Here's how the part is built. I have some questions about the finished solid (model axes, mm). Give positions to 0.01 mm unless a question says otherwise; leave off trailing zeros. Write each loop counter-clockwise with the first axis right and the second up, starting at its lowest first coordinate (ties: lowest second). Pieces come first, ordered by that corner, then holes. Notation, with made-up numbers: (33, 4) - (76, 4) arc R14 cw to (76, 24) - close; hole circle Ø8 at (39.25, -29). An arc over 180 degrees is marked (long way). One line per item, written item: value. Start each with the question number.
1) Imagine slicing it at A-A on z = 50. Write out the boundary of the cut face in (x, y), plus the area to 3 significant figures.
2) I'm going to push a flat-ended pin straight in: P1, Ø6, axis at x = -79.4, z = 50, coming from the +Y side. Where does the tip first touch, or does it pass through?
3) Imagine slicing it at B-B on x = 79.4. Write out the boundary of the cut face in (y, z), plus the area to 3 significant figures.
4) Please list where these lines run through material, in increasing order: L1, parallel to X at y = -4.5, z = 50; L2, parallel to Z at x = -79.4, y = -3.5. Write a range as [from, to].
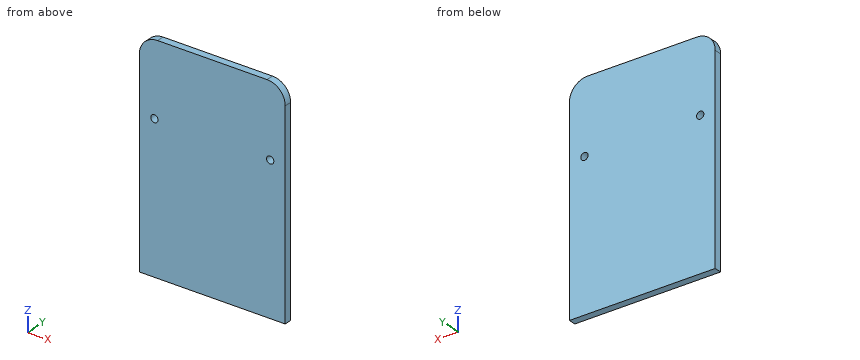
from build123d import *

# Parameters (mm, degrees)
BOSS_EXTRUDE1_DEPTH = 10
SKETCH2_R           = 5
CUT_EXTRUDE1_DEPTH  = 11


with BuildPart() as part:
    # Sketch1 → Boss-Extrude1 (new body)
    with BuildSketch(Plane(origin=(0, 0, 0), x_dir=(1, 0, 0), z_dir=(0, 1, 0))):
        with BuildLine():
            Line((-100, 150), (100, 150))
            Line((100, 150), (100, -125))
            ThreePointArc((100, -125), (92.67766953, -142.67766953), (75, -150))
            Line((75, -150), (-75, -150))
            ThreePointArc((-75, -150), (-92.67766953, -142.67766953), (-100, -125))
            Line((-100, -125), (-100, 150))
        make_face()
    extrude(amount=-BOSS_EXTRUDE1_DEPTH)

    # Sketch2 → Cut-Extrude1 (cut, through all)
    with BuildSketch(Plane(origin=(0, 0, 0), x_dir=(1, 0, 0), z_dir=(0, 1, 0))):
        with Locations((-79.4, -50)):
            Circle(SKETCH2_R)
        with Locations((79.4, -50)):
            Circle(SKETCH2_R)
    extrude(amount=-CUT_EXTRUDE1_DEPTH, mode=Mode.SUBTRACT)


solid = part.part
Numbers:
1. outline: (-100, -10) - (-84.4, -10) - (-84.4, 0) - (-100, 0) - close; (-74.4, -10) - (74.4, -10) - (74.4, 0) - (-74.4, 0) - close; (84.4, -10) - (100, -10) - (100, 0) - (84.4, 0) - close
1. area: 1,800 mm^2
2. P1: through
3. outline: (-10, -150) - (0, -150) - (0, 45) - (-10, 45) - close; (-10, 55) - (0, 55) - (0, 149.61) - (-10, 149.61) - close
3. area: 2,900 mm^2
4. L1: [-100, -84.4], [-74.4, 74.4], [84.4, 100]
4. L2: [-150, 45], [55, 149.61]
